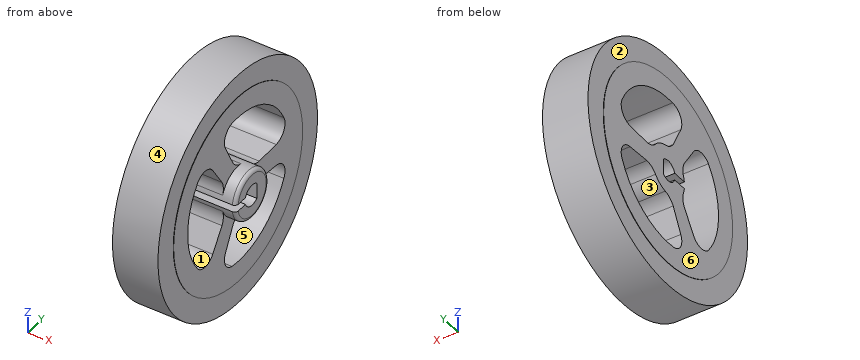
```python
from build123d import *

# Parameters (mm, degrees)
RESSALTO_EXTRUS_O1_DEPTH      = 5.3
RESSALTO_EXTRUS_O1_DEPTH_BACK = 3.3
ESBO_O1_3_R                   = 13.75
RESSALTO_EXTRUS_O2_DEPTH      = 3.3
FILETE2_R                     = 0.5
ESBO_O2_R                     = 17
ESBO_O2_R_2                   = 13.75
RESSALTO_EXTRUS_O3_DEPTH      = 3.25


with BuildPart() as part:
    # Esboço1 → Ressalto-extrusão1 (new, two sides: drawn at the far end of the back side and taken through both)
    with BuildSketch(Plane(origin=(0, 0, 0), x_dir=(0, 0, -1), z_dir=(1, 0, 0)).offset(-RESSALTO_EXTRUS_O1_DEPTH_BACK)):
        with BuildLine():
            ThreePointArc((0.5, -1.414213562), (1.4531398, -0.37200097), (1.118033989, 1))
            Line((1.118033989, 1), (-1.118033989, 1))
            ThreePointArc((-1.118033989, 1), (-1.4531398, -0.37200097), (-0.5, -1.414213562))
            Line((-0.5, -1.414213562), (-0.5, -3.464101615))
            ThreePointArc((-0.5, -3.464101615), (0, 3.5), (0.5, -3.464101615))
            Line((0.5, -3.464101615), (0.5, -1.414213562))
        make_face()
    extrude(amount=RESSALTO_EXTRUS_O1_DEPTH + RESSALTO_EXTRUS_O1_DEPTH_BACK)

    # Esboço1<3> → Ressalto-extrusão2 (add, symmetric)
    with BuildSketch(Plane(origin=(0, 0, 0), x_dir=(0, 0, -1), z_dir=(1, 0, 0))):
        Circle(ESBO_O1_3_R)
        with BuildLine():
            ThreePointArc((3.446771953, 0.608081497), (3.031088913, -1.75), (1.196771953, -3.28903282))
            ThreePointArc((1.196771953, -3.28903282), (2.228560776, -3.144612223), (3.229618168, -3.433280857))
            Line((3.229618168, -3.433280857), (6.244929793, -5.410607922))
            ThreePointArc((6.244929793, -5.410607922), (7.143531761, -6.946693722), (6.462297299, -8.590763273))
            ThreePointArc((6.462297299, -8.590763273), (0, -10.75), (-6.462297299, -8.590763273))
            ThreePointArc((-6.462297299, -8.590763273), (-7.143531761, -6.946693722), (-6.244929793, -5.410607922))
            Line((-6.244929793, -5.410607922), (-3.229618168, -3.433280857))
            ThreePointArc((-3.229618168, -3.433280857), (-2.228560776, -3.144612223), (-1.196771953, -3.28903282))
            ThreePointArc((-1.196771953, -3.28903282), (-3.031088913, -1.75), (-3.446771953, 0.608081497))
            ThreePointArc((-3.446771953, 0.608081497), (-3.837594458, -0.357684134), (-4.588117525, -1.08029095))
            Line((-4.588117525, -1.08029095), (-7.808188807, -2.702963885))
            ThreePointArc((-7.808188807, -2.702963885), (-9.742921821, -2.628468224), (-10.707946608, -0.949936544))
            ThreePointArc((-10.707946608, -0.949936544), (-9.309773091, 5.375), (-4.531304125, 9.748322057))
            ThreePointArc((-4.531304125, 9.748322057), (-2.595140656, 9.751851916), (-1.563259014, 8.113571807))
            Line((-1.563259014, 8.113571807), (-1.358499357, 4.513571807))
            ThreePointArc((-1.358499357, 4.513571807), (-1.609033682, 3.502296357), (-2.25, 2.680951324))
            ThreePointArc((-2.25, 2.680951324), (0, 3.5), (2.25, 2.680951324))
            ThreePointArc((2.25, 2.680951324), (1.609033682, 3.502296357), (1.358499357, 4.513571807))
            Line((1.358499357, 4.513571807), (1.563259014, 8.113571807))
            ThreePointArc((1.563259014, 8.113571807), (2.595140656, 9.751851916), (4.531304125, 9.748322057))
            ThreePointArc((4.531304125, 9.748322057), (9.396801436, 5.221362156), (10.670967882, -1.301131991))
            ThreePointArc((10.670967882, -1.301131991), (9.587779116, -2.713133117), (7.808188807, -2.702963885))
            Line((7.808188807, -2.702963885), (4.588117525, -1.08029095))
            ThreePointArc((4.588117525, -1.08029095), (3.837594458, -0.357684134), (3.446771953, 0.608081497))
        make_face(mode=Mode.SUBTRACT)
    extrude(amount=RESSALTO_EXTRUS_O2_DEPTH, both=True)

    # Filete2
    filete2_edges = [part.edges().sort_by_distance(p)[0] for p in [
        (5.3, 3.5, 0),
    ]]
    fillet(filete2_edges, radius=FILETE2_R)

    # Esboço2 → Ressalto-extrusão3 (add, symmetric)
    with BuildSketch(Plane(origin=(0, 0, 0), x_dir=(0, 0, -1), z_dir=(1, 0, 0))):
        with Locations(Location((0, 0, 0), (0, 0, 180))):
            Circle(ESBO_O2_R)
        Circle(ESBO_O2_R_2, mode=Mode.SUBTRACT)
    extrude(amount=RESSALTO_EXTRUS_O3_DEPTH, both=True)


solid = part.part
```
Check sheet for the modelled part. Datum: model origin and axes. Units: mm. Face numbers are marked on the shaded views. A direction names the side the tool comes from. Round coordinates to 2 decimals unless told otherwise and drop trailing zeros. Loops run counter-clockwise (first coordinate to the right, second up) from the corner with the lowest first, then second, coordinate; pieces in that order, holes last. Notation, with made-up numbers: (7, -34) -> (17, -34) arc R19 ccw to (17, -9) -> close; hole circle Ø5 at (-17, -10). An arc over 180 degrees is marked (long way). Answer in a Markdown table with one row per item.
Q1. Sectioned sample at B-B on y = -4. Enter the section's corners in (x, z).
Data:
| item | result |
|---|---|
| outline | (-3.3, -13.16) -> (-3.25, -13.16) -> (-3.25, -16.52) -> (3.25, -16.52) -> (3.25, -13.16) -> (3.3, -13.16) -> (3.3, -4.09) -> (-3.3, -4.09) -> close; (-3.3, 4.09) -> (3.3, 4.09) -> (3.3, 13.16) -> (3.25, 13.16) -> (3.25, 16.52) -> (-3.25, 16.52) -> (-3.25, 13.16) -> (-3.3, 13.16) -> close |
Q2. Go/stop test with flat-tipped pins: P1, Ø1.6, axis at x = -1, y = -2.5, coming from the -Z side; P2, Ø2, axis at y = 5, z = 1.5, coming from the +X side; P3, Ø2.5, axis at x = 0.5, y = -2, coming from the +Z side. Record where each tip stops, or that it passes through.
Data:
| item | result |
|---|---|
| P1 | stops at z = -16.91 |
| P2 | stops at x = 3.3 |
| P3 | stops at z = 16.98 |
Q3. Set-up check for the marked faces 1, 2 and 3: record each of +Z, -Z, +X, -X, +Y, -Y from which the full face is reachable in a straight line by a thin tool's end or side.
Data:
| item | result |
|---|---|
| face 1 | +X, -X |
| face 2 | -X |
| face 3 | +X |
Q4. Sectioned sample at C-C on x = 4.25. Enter the section's corners in (y, z).
Data:
| item | result |
|---|---|
| outline | (-3.46, -0.5) arc R3.5 ccw (long way) to (-3.46, 0.5) -> (-1.41, 0.5) arc R1.5 cw to (1, 1.12) -> (1, -1.12) arc R1.5 cw to (-1.41, -0.5) -> close |
Q5. Thickness scan on L1, parallel to Z at x = -1, y = 4.5; L2, parallel to Z at x = -2, y = 3.5; L3, parallel to Y at x = -2, z = 2. Record the ranges inside material, lowest first.
Data:
| item | result |
|---|---|
| L1 | z = -16.39 to -9.76, -1.36 to 1.36, 9.76 to 16.39 |
| L2 | z = -16.64 to -10.16, -1.61 to 1.61, 10.16 to 16.64 |
| L3 | y = -16.88 to -10.56, -3.14 to 2.92, 9.25 to 16.88 |
Q6. Sectioned sample at A-A on z = 0. Enter the section's corners in (x, y).
Data:
| item | result |
|---|---|
| outline | (-3.3, -13.75) -> (-3.25, -13.75) -> (-3.25, -17) -> (3.25, -17) -> (3.25, -13.75) -> (3.3, -13.75) -> (3.3, -10.75) -> (-3.3, -10.75) -> close; (-3.3, 1) -> (5.3, 1) -> (5.3, 3) arc R0.5 ccw to (4.8, 3.5) -> (3.3, 3.5) -> (3.3, 13.75) -> (3.25, 13.75) -> (3.25, 17) -> (-3.25, 17) -> (-3.25, 13.75) -> (-3.3, 13.75) -> close |
Q7. Release check for a two-part mould opening along Z. For the marked faces 4, 5 and 6 record: released by +Z, released by -Z, zero draft, split by the parting line, or undercut.
Data:
| item | result |
|---|---|
| face 4 | split by the parting line |
| face 5 | undercut |
| face 6 | zero draft |
Q8. Sectioned sample at D-D on y = 5.5. Enter the section's corners in (x, z), then the cut area to 3 significant figures.
Data:
| item | result |
|---|---|
| outline | (-3.3, -12.6) -> (-3.25, -12.6) -> (-3.25, -16.09) -> (3.25, -16.09) -> (3.25, -12.6) -> (3.3, -12.6) -> (3.3, -9.24) -> (-3.3, -9.24) -> close; (-3.3, -1.41) -> (3.3, -1.41) -> (3.3, 1.41) -> (-3.3, 1.41) -> close; (-3.3, 9.24) -> (3.3, 9.24) -> (3.3, 12.6) -> (3.25, 12.6) -> (3.25, 16.09) -> (-3.25, 16.09) -> (-3.25, 12.6) -> (-3.3, 12.6) -> close |
| area | 108 mm^2 |
